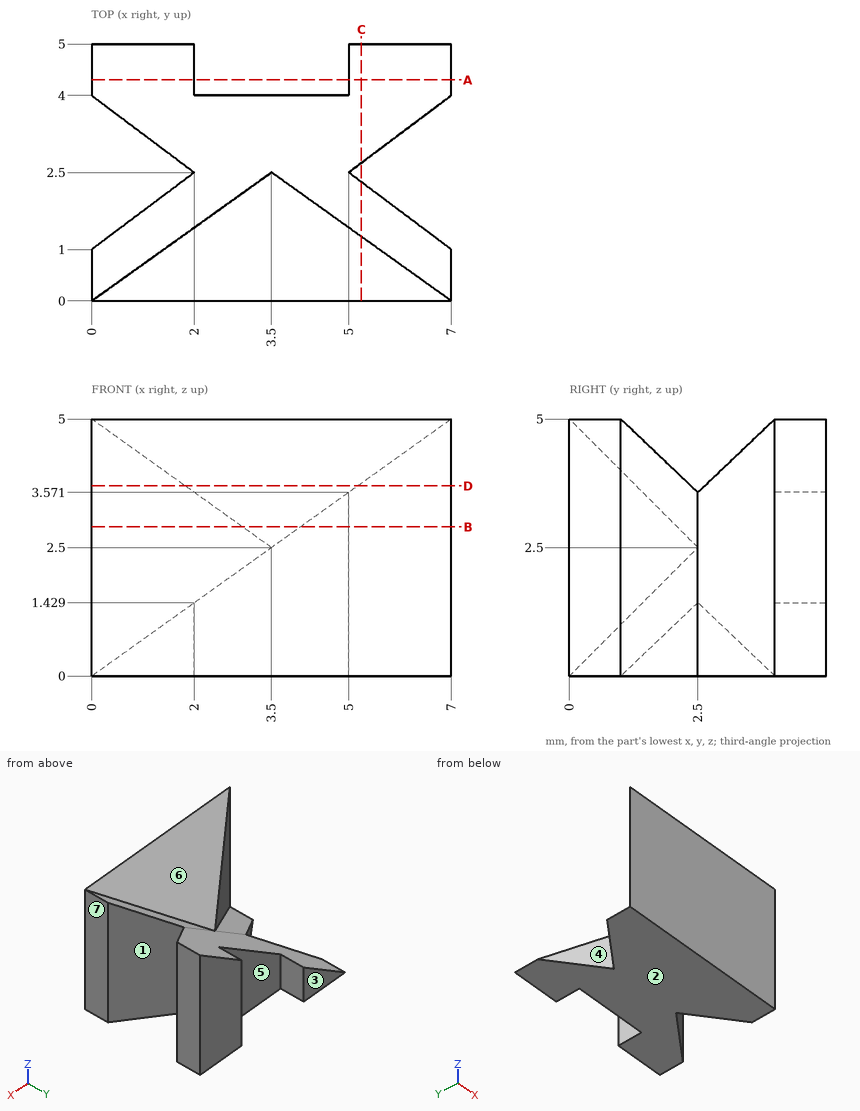
Job drawing, mm, ordinate dimensions from the low corner. One solid piece. A direction names the side the tool comes from. Coordinates: 2 decimals unless noted, no trailing zeros. Order: outer loops, then holes, each group sorted by start corner. A loop starts at its lowest first (then second) coordinate and runs counter-clockwise, first axis right, second up. Notation, with made-up numbers: (27.25, -8) -> (36.25, -8) arc R22 ccw to (36.25, 17) -> close; hole circle Ø10 at (-2.75, 10.25). An arc over 180 degrees is marked (long way). Answer in a Markdown table with one row per item. Add a question column.
Q1. Band-saw the part on B-B, the plane z = 2.9. List the corners of the cut face in (x, y).
Q2. Drop flat-ended pins along their axis: pin 1 (1.5 mm diameter, centred on y = 1.5, z = 2, fed in from +X); pin 2 (0.5 mm diameter, centred on y = 4.5, z = 2.5, fed in from -X); pin 3 (1.5 mm diameter, centred on x = 4, z = 1.5, fed in from +Y); pin 4 (2 mm diameter, centred on x = 1, y = 2, fed in from +Z). Give the stop position or say it passes through.
Q3. Band-saw the part on D-D, the plane z = 3.7. List the corners of the cut face in (x, y) (1 decimal), then the cut area to 3 significant figures.
Q4. Mould opens along Y. For the marked faces 1, 2, 3 and 4 say: +Y half, -Y half, draft (parallel to the pull), parting line (faces both ways), or undercut.
Q5. Which spindle directions (+Z, -Z, +X, -X, +Y, -Y) get a long thin tool onto all of the face, cutting with end or side? Do the marked faces 5, 6 and 7. Say none if no direction does.
Q6. Band-saw the part on C-C, the plane x = 5.25. List the corners of the cut face in (y, z), then the cut area to 3 significant figures.
Q7. Band-saw the part on A-A, the plane y = 4.3. List the corners of the cut face in (x, z).
Q8. Wall check: line 1 along Y through (x, z) = (3.25, 2.2); line 2 along Z through (x, y) = (2, 2); line 3 along X through (y, z) = (4.5, 0.6). Give the ranges that are in metal, low to high. Write a range as [from, to].
Answers follow:
| question | item | result |
|---|---|---|
| 1 | outline | (0, 0) -> (7, 0) -> (7, 1) -> (5, 2.5) -> (7, 4) -> (7, 5) -> (5, 5) -> (5, 4) -> (4.06, 4) -> (4.06, 2.1) -> (2.94, 2.1) -> close |
| 2 | pin 1 | x = 7 |
| 2 | pin 2 | x = 5 |
| 2 | pin 3 | y = 4 |
| 2 | pin 4 | z = 1.43 |
| 3 | outline | (0, 0) -> (7, 0) -> (7, 1) -> (5.2, 2.4) -> (5.2, 1.3) -> (1.8, 1.3) -> close; (5.2, 2.6) -> (7, 4) -> (7, 5) -> (5.2, 5) -> close |
| 3 | area | 11.7 mm^2 |
| 4 | face 1 | undercut |
| 4 | face 2 | draft |
| 4 | face 3 | +Y half |
| 4 | face 4 | undercut |
| 5 | face 5 | +Z, -Z, +Y |
| 5 | face 6 | +Z, -X, +Y |
| 5 | face 7 | +Z, -Z, +X, +Y, -Y |
| 6 | outline | (0, 0) -> (2.31, 0) -> (2.31, 3.75) -> (1.25, 3.75) -> (0, 5) -> close; (2.69, 0) -> (5, 0) -> (5, 3.75) -> (2.69, 3.75) -> close |
| 6 | area | 18.1 mm^2 |
| 7 | outline | (0, 0) -> (2, 0) -> (2, 1.43) -> close; (5, 0) -> (7, 0) -> (7, 5) -> (5, 3.57) -> close |
| 8 | line 1 | [0, 4] |
| 8 | line 2 | [0, 1.43] |
| 8 | line 3 | [0.84, 2], [5, 7] |
